```python
from build123d import *

# Parameters (mm, degrees)
SKETCH2_R           = 100
SKETCH2_R_2         = 98
BOSS_EXTRUDE2_DEPTH = 50
BOSS_EXTRUDE3_DEPTH = 50
CIRPATTERN1_COUNT   = 20
SKETCH7_R           = 98
SKETCH7_R_2         = 96
BOSS_EXTRUDE5_DEPTH = 5
SKETCH14_W          = 10
SKETCH14_H          = 7
BOSS_EXTRUDE8_DEPTH = 10
SKETCH15_R          = 2.5
CUT_EXTRUDE3_DEPTH  = 10
CIRPATTERN6_COUNT   = 6


with BuildPart() as part:
    # Sketch2 → Boss-Extrude2 (new, symmetric)
    with BuildSketch(Plane.XY):
        Circle(SKETCH2_R)
        Circle(SKETCH2_R_2, mode=Mode.SUBTRACT)
    extrude(amount=BOSS_EXTRUDE2_DEPTH, both=True)

    # Sketch4 → Boss-Extrude3 (add, symmetric)
    with BuildSketch(Plane.XY):
        Polygon((0, 101.99718746), (-0.75, 101.99718746), (-0.75, 99.99718746), (0.75, 99.99718746), (0.75, 101.99718746), align=None)
    boss_extrude3 = extrude(amount=BOSS_EXTRUDE3_DEPTH, both=True)

    # CirPattern1: Boss-Extrude3 ×20 about axis
    cirpattern1_axis = Axis((0, 0, 0), (0, 0, 1))
    for i in range(1, CIRPATTERN1_COUNT):
        add(boss_extrude3.rotate(cirpattern1_axis, i * 360 / CIRPATTERN1_COUNT))

    # Sketch7 → Boss-Extrude5 (add, symmetric)
    with BuildSketch(Plane.XY.offset(20)):
        Circle(SKETCH7_R)
        Circle(SKETCH7_R_2, mode=Mode.SUBTRACT)
    extrude(amount=BOSS_EXTRUDE5_DEPTH, both=True)

    # Sketch14 → Boss-Extrude8 (add)
    with BuildSketch(Plane.XY.offset(25)):
        with Locations((0, 92.5)):
            Rectangle(SKETCH14_W, SKETCH14_H)
    boss_extrude8 = extrude(amount=-BOSS_EXTRUDE8_DEPTH)

    # Sketch15 → Cut-Extrude3 (cut)
    with BuildSketch(Plane.XY.offset(25)):
        with Locations((0, 92.5)):
            Circle(SKETCH15_R)
    cut_extrude3 = extrude(amount=-CUT_EXTRUDE3_DEPTH, mode=Mode.SUBTRACT)

    # CirPattern6: Boss-Extrude8, Cut-Extrude3 ×6 about axis
    cirpattern6_axis = Axis((0, 0, 0), (0, 0, 1))
    add([boss_extrude8.rotate(cirpattern6_axis, i * 360 / CIRPATTERN6_COUNT) for i in range(1, CIRPATTERN6_COUNT)])
    add([cut_extrude3.rotate(cirpattern6_axis, i * 360 / CIRPATTERN6_COUNT) for i in range(1, CIRPATTERN6_COUNT)], mode=Mode.SUBTRACT)


solid = part.part
```
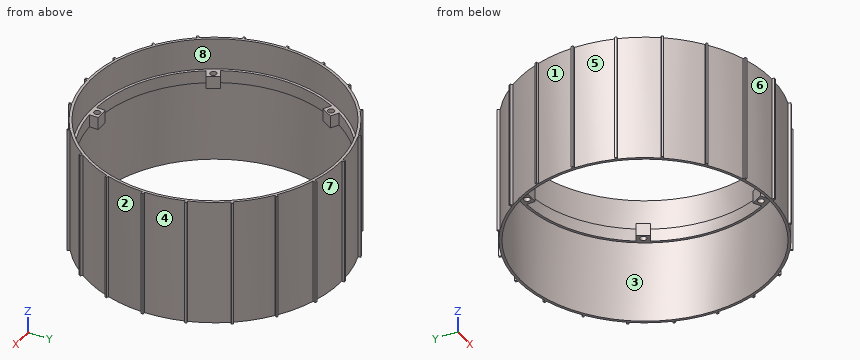
Work out the finished part from the listing and answer in its coordinate system (mm). Face numbers are marked on the shaded views. A direction names the side the tool comes from. Give positions to 0.01 mm unless a question says otherwise; leave off trailing zeros. Loops run counter-clockwise (first coordinate to the right, second up) from the corner with the lowest first, then second, coordinate; pieces in that order, holes last. Notation, with made-up numbers: (-17.75, -37.5) -> (7.25, -37.5) arc R18 ccw to (7.25, -9.5) -> close; hole circle Ø9 at (59.25, 38). An arc over 180 degrees is marked (long way). Write item = value, one per line. Start each with the question number.
(1) Find the intervals of material crossed by probe 1 along X at (y, z) = (46, 17); probe 2 along X at (y, z) = (69.5, 2); probe 3 along X at (y, z) = (51, -38), in increasing order. Write a range as from..to.
(2) Find section A-A on x = -17. Give the vertices of the cut face in (y, z), and give its area (3 significant figures).
(3) Given pin 1 Ø1 at (y, z) = (101.5, 14.5) entering from -X; pin 2 Ø1 at (x, z) = (-101, -3) entering from +Y; pin 3 Ø2 at (x, z) = (101.5, 16) entering from +Y, each flat-ended and moving along its own axis, determine where each tip first touches the part or whether it passes through.
(4) The mould has two halves that part along X. Classify the marked faces 1, 2 and 3: +X half, -X half, draft (parallel to the pull), parting line (faces both ways), or undercut.
(5) Which of the six approach directions +Z, -Z, +X, -X, +Y, -Y give full straight-line access (tool end or side, diameter ignored) to the marked faces 4, 5, 6, 7 and 8?
(6) Find section C-C on z = 21.5. Give the number of separate pieces and of enclosed holes in the cut face, and give its area (3 significant figures).
From the geometry:
q1.probe_1 = -88.79..-82.59, -77.62..-76.21, 76.21..77.62, 82.59..88.79
q1.probe_2 = -71.9..-69.09, 69.09..71.9
q1.probe_3 = -86.02..-83.68, 83.68..86.02
q2.outline = (-98.54, -50) -> (-96.51, -50) -> (-96.51, 15) -> (-94.48, 15) -> (-94.48, 25) -> (-96.51, 25) -> (-96.51, 50) -> (-98.54, 50) -> close; (94.48, 15) -> (96.51, 15) -> (96.51, -50) -> (98.54, -50) -> (98.54, 50) -> (96.51, 50) -> (96.51, 25) -> (94.48, 25) -> close
q2.area = 447 mm^2
q3.pin_1 = -0.75
q3.pin_2 = 0.75
q3.pin_3 = 0.75
q4.face_1 = -X half
q4.face_2 = +X half
q4.face_3 = undercut
q5.face_4 = +Z, -Z, +X
q5.face_5 = +Z, -Z, -X
q5.face_6 = +Z, -Z, -Y
q5.face_7 = +Z, -Z, +Y
q5.face_8 = +Z
q6.separate_pieces = 1
q6.enclosed_holes = 7
q6.area = 2,820 mm^2
